Design review of the part built by this model. Coordinates are the model's own, in mm. Coordinates: 2 decimals unless noted, no trailing zeros. Write each loop counter-clockwise with the first axis right and the second up, starting at its lowest first coordinate (ties: lowest second). Pieces come first, ordered by that corner, then holes.
Q1. To check wall thickness, follow probe 1 along X at (y, z) = (102, 0); probe 2 along Z at (x, y) = (-0.25, 89). State the ranges of each line that lie inside material, in increasing order.
Q2. Add section A-A, the plane y = 74. Give the boundary of the cut face in (x, z).
Q3. Clearance check with flat-ended pins moving along their axes: pin 1 Ø0.5 at (y, z) = (19, 3) entering from +X; pin 2 Ø3 at (x, y) = (0.5, 46) entering from -Z; pin 3 Ø0.9 at (y, z) = (53, 3) entering from -X; pin 4 Ø1 at (x, y) = (3, 93.5) entering from +Z. State where each tip first meets the part, or that it passes through.
Q4. The part is to be moulded in two halves that separate along X. For faces 1 (the face through (2.343, -12.878, 1.494)), 2 (the face through (1.4, 66.2, -2.6)), 3 (the face through (-1.092, -12.522, -1.425)), 4 (the face through (-1, -25.4, 0)), say which applies: +X half, -X half, draft (parallel to the pull), parting line (faces both ways), or undercut.
from build123d import *

# Parameters (mm, degrees)
F0_R          = 3.96875
F0_R_2        = 2.95275
F1_DEPTH      = 134.366
F3_DEPTH      = 3.96975
F3_DEPTH_BACK = 3.96975
F7_R          = 0.79375
F8_DEPTH      = 12.7
F9_DEPTH      = 3.9697501215


# Not quite as in the source:
# - the program builds the solid bodies; features that only make, move or delete a surface that nothing else refers to are left out


with BuildPart() as f1:
    # F0 (on Front) → F1 (new body)
    with BuildSketch(Plane.XZ):
        Circle(F0_R)
        Circle(F0_R_2, mode=Mode.SUBTRACT)
    extrude(amount=-F1_DEPTH)

    # F2 (on Top) → F3 (cut, two sides)
    with BuildSketch(Plane.XY) as f3_sk:
        with BuildLine():
            ThreePointArc((1.143, 31.75), (0, 32.893), (-1.143, 31.75))
            Line((-1.143, 31.75), (-1.143, 12.7))
            ThreePointArc((-1.143, 12.7), (0, 11.557), (1.143, 12.7))
            Line((1.143, 12.7), (1.143, 31.75))
        make_face()
    extrude(amount=F3_DEPTH, mode=Mode.SUBTRACT)
    extrude(f3_sk.sketch, amount=-F3_DEPTH_BACK, mode=Mode.SUBTRACT)

    # F5 (on Right) → F6 (revolve)
    with BuildSketch(Plane.YZ):
        Polygon((0, 3.96875), (-25.4, 1.6208575107), (-25.4, 0.6048575107), (0, 2.95275), align=None)
    revolve(axis=Axis((0, -12.7, 0), (0, 1, 0)))

    # F7 (on Right) → F8 (cut, symmetric)
    with BuildSketch(Plane.YZ):
        with Locations((3.175, 0)):
            Circle(F7_R)
    extrude(amount=F8_DEPTH, both=True, mode=Mode.SUBTRACT)

    # F4 (on Top) → F9 (cut, through all)
    with BuildSketch(Plane.XY):
        with BuildLine():
            ThreePointArc((1.27, 62.165913868), (0, 63.435913868), (-1.27, 62.165913868))
            Line((-1.27, 62.165913868), (-1.27, 43.115913868))
            ThreePointArc((-1.27, 43.115913868), (-1.1164401975, 42.5105534089), (-0.6928956136, 42.0515851271))
            Line((-0.6928956136, 42.0515851271), (-0.6928956136, 31.9918245077))
            Line((-0.6928956136, 31.9918245077), (0.6928956136, 31.9918245077))
            Line((0.6928956136, 31.9918245077), (0.6928956136, 42.0515851271))
            ThreePointArc((0.6928956136, 42.0515851271), (1.1164401975, 42.5105534089), (1.27, 43.115913868))
            Line((1.27, 43.115913868), (1.27, 62.165913868))
        make_face()
    extrude(amount=F9_DEPTH, mode=Mode.SUBTRACT)


solid = f1.part
Here are the results:
1. probe 1: x = -3.97 to -2.95, 2.95 to 3.97
1. probe 2: z = -3.96 to -2.94, 2.94 to 3.96
2. outline: circle Ø7.94 at (0, 0); hole circle Ø5.91 at (0, 0)
3. pin 1: stops at x = 2.86
3. pin 2: stops at z = -3.97
3. pin 3: stops at x = -3.04
3. pin 4: stops at z = 3.08
4. face 1: parting line
4. face 2: undercut
4. face 3: undercut
4. face 4: draft
